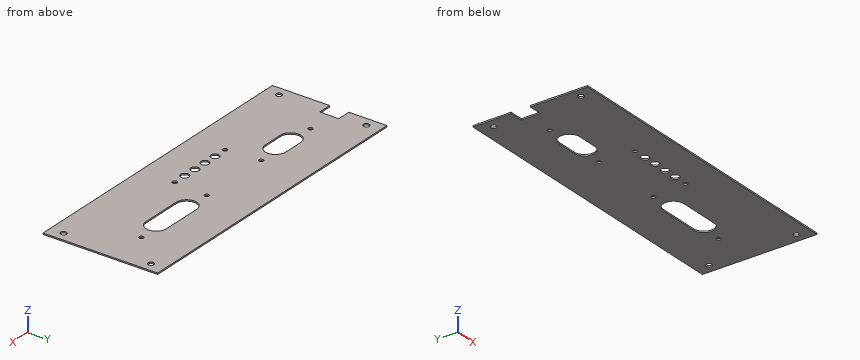
```python
from build123d import *

# Parameters (mm, degrees)
SKETCH_1_W          = 228
SKETCH_1_H          = 84
SKETCH_1_R          = 2.15
EXTRUDE_1_DEPTH     = 1
SKETCH_4_R          = 1.6
SKETCH_4_W          = 14.464145402
SKETCH_4_H          = 14
CUT_EXTRUDE_2_DEPTH = 1
SKETCH_5_R          = 1.7
SKETCH_5_R_2        = 3
CUT_EXTRUDE_3_DEPTH = 10


with BuildPart() as part:
    # Эскиз1 → Вытянуть1 (new body)
    with BuildSketch(Plane.XY):
        Rectangle(SKETCH_1_W, SKETCH_1_H)
        with Locations((107, 32)):
            Circle(SKETCH_1_R, mode=Mode.SUBTRACT)
        with Locations(Location((-107, 32, 0), (0, 0, 180))):
            Circle(SKETCH_1_R, mode=Mode.SUBTRACT)
        with Locations((-107, -32)):
            Circle(SKETCH_1_R, mode=Mode.SUBTRACT)
        with Locations(Location((107, -32, 0), (0, 0, 180))):
            Circle(SKETCH_1_R, mode=Mode.SUBTRACT)
    extrude(amount=EXTRUDE_1_DEPTH)

    # Эскиз4 → Вырез-Вытянуть2 (cut)
    with BuildSketch(Plane.XY.offset(1)):
        with Locations((19, 8)):
            Circle(SKETCH_4_R)
        with Locations((84, 8)):
            Circle(SKETCH_4_R)
        with Locations((-84, 8)):
            Circle(SKETCH_4_R)
        with Locations((-35, 8)):
            Circle(SKETCH_4_R)
        with BuildLine():
            Line((36.5, 13.5), (66.5, 13.5))
            ThreePointArc((66.5, 13.5), (74, 6), (66.5, -1.5))
            Line((66.5, -1.5), (36.5, -1.5))
            ThreePointArc((36.5, -1.5), (29, 6), (36.5, 13.5))
        make_face()
        with BuildLine():
            Line((-67, 13.5), (-52, 13.5))
            ThreePointArc((-52, 13.5), (-44.5, 6), (-52, -1.5))
            Line((-52, -1.5), (-67, -1.5))
            ThreePointArc((-67, -1.5), (-74.5, 6), (-67, 13.5))
        make_face()
        with Locations((-111.232072701, 7)):
            Rectangle(SKETCH_4_W, SKETCH_4_H)
    extrude(amount=-CUT_EXTRUDE_2_DEPTH, mode=Mode.SUBTRACT)

    # Эскиз5 → Вырез-Вытянуть3 (cut)
    with BuildSketch(Plane.XY.offset(1)):
        with Locations((-33, -17)):
            Circle(SKETCH_5_R)
        with Locations((17, -17)):
            Circle(SKETCH_5_R)
        with Locations((7, -17)):
            Circle(SKETCH_5_R_2)
        with Locations((-3, -17)):
            Circle(SKETCH_5_R_2)
        with Locations((-13, -17)):
            Circle(SKETCH_5_R_2)
        with Locations((-23, -17)):
            Circle(SKETCH_5_R_2)
    extrude(amount=-CUT_EXTRUDE_3_DEPTH, mode=Mode.SUBTRACT)


solid = part.part
```
Work out the finished part from the listing and answer in its coordinate system (mm). Coordinates: 2 decimals unless noted, no trailing zeros. Write each loop counter-clockwise with the first axis right and the second up, starting at its lowest first coordinate (ties: lowest second). Pieces come first, ordered by that corner, then holes.
Q1. A cutting plane is placed at A-A, the plane x = -3. Give the vertices of the cut face in (y, z), then the cut area to 3 significant figures.
Q2. Each of these flat-tipped pins is pushed along its axis until it touches: pin 1 Ø2 at (x, y) = (55.5, 33.5) entering from -Z; pin 2 Ø0.5 at (y, z) = (8, 0.5) entering from -X. Where does it stop, or does it pass through?
Q3. Find the intervals of material crossed by line 1 (Y direction, x = 84, z = 0.7); line 2 (Y direction, x = -3, z = 0.45); line 3 (X direction, y = -33, z = 0.25), in increasing order.
Q4. A cutting plane is placed at B-B, the plane y = 3. Give the vertices of the cut face in (x, z).
Q5. A cutting plane is placed at C-C, the plane z = 0.35. State how many separate pieces and enclosed holes the cut face has, then the cut area to 3 significant figures.
Q6. A cutting plane is placed at D-D, the plane x = 54.5. Give the vertices of the cut face in (y, z), then the cut area to 3 significant figures.
Findings below:
1. outline: (-42, 0) - (-20, 0) - (-20, 1) - (-42, 1) - close; (-14, 0) - (42, 0) - (42, 1) - (-14, 1) - close
1. area: 78.0 mm2
2. pin 1: stops at z = 0
2. pin 2: stops at x = -104
3. line 1: y = -42 to 6.4, 9.6 to 42
3. line 2: y = -42 to -20, -14 to 42
3. line 3: x = -114 to -108.9, -105.1 to 105.1, 108.9 to 114
4. outline: (-104, 0) - (-73.87, 0) - (-73.87, 1) - (-104, 1) - close; (-45.13, 0) - (29.63, 0) - (29.63, 1) - (-45.13, 1) - close; (73.37, 0) - (114, 0) - (114, 1) - (73.37, 1) - close
5. separate pieces: 1
5. enclosed holes: 16
5. area: 17,800 mm2
6. outline: (-42, 0) - (-1.5, 0) - (-1.5, 1) - (-42, 1) - close; (13.5, 0) - (42, 0) - (42, 1) - (13.5, 1) - close
6. area: 69.0 mm2
